Part model, mm, in its own coordinate system. Face numbers are marked on the shaded views. A direction names the side the tool comes from. Give positions to 0.01 mm unless a question says otherwise; leave off trailing zeros. Loops run counter-clockwise (first coordinate to the right, second up) from the corner with the lowest first, then second, coordinate; pieces in that order, holes last. Notation, with made-up numbers: M 89,89.25 L 128,89.25 A29 cw 128,124.25 Z; hole C 29.5,70.25 d9. An arc over 180 degrees is marked long. Put each result on its own line as item: value. Start each with the question number.
Autodesk Inventor part; units mm, degrees
ref_plane "YZ Plane" through (0, 0, 0) normal (1, 0, 0) x (0, 1, 0)
ref_plane "XZ Plane" through (0, 0, 0) normal (0, 1, 0) x (-1, 0, 0)
ref_plane "XY Plane" through (0, 0, 0) normal (0, 0, 1) x (1, 0, 0)
sketch "Sketch1" plane through (0, 0, 0) normal (1, 0, 0) x (0, 1, 0)
  line L0 (16, 0) -> (-16, 0)
  line L1 (16, 0) -> (-16, 0) construction
  line L2 (21.5, 0) -> (16, 0)
  line L3 (21.9436, -96.7485) -> (36.9412, -122.057)
  line L4 (21.5, -4) -> (21.5, -95.1299)
  line L5 (21.5, -95.1299) -> (21.9436, -96.7485)
  line L6 (37.5, -124.0962) -> (37.5, -137.065)
  line L7 (36.9412, -122.057) -> (37.5, -123)
  line L8 (37.5, -123) -> (37.5, -124.0962)
  arc A0 (37.5, -124.0962) -> (36.9412, -122.057) centre (33.5, -124.0962) ccw construction
  line L9 (-16, 0) -> (-20.5, 0)
  line L10 (-20.5, 0) -> (-20.5, -95.1299)
  line L11 (-20.5, -95.1299) -> (-20.5, -4) construction
  line L12 (-20.5, -7.5) -> (-159.2, -7.5)
  line L13 (-159.2, -7.5) -> (-159.2, -52.5)
  line L14 (-159.2, -52.5) -> (-20.5, -52.5)
  line L15 (-73.4, -7.5) -> (-107.4, -7.5) construction
  line L16 (-73.4, -52.5) -> (-107.4, -52.5) construction
  line L17 (-159.2, -35.5) -> (-159.2, -24.5) construction
  line L18 (-35.9412, -122.057) -> (-20.9436, -96.7485)
  line L19 (-20.5, -95.1299) -> (-20.9436, -96.7485)
  line L20 (-36.5, -137.065) -> (-36.5, -124.0962)
  arc A1 (-35.9412, -122.057) -> (-36.5, -124.0962) centre (-32.5, -124.0962) ccw construction
  line L21 (-35.9412, -122.057) -> (-36.5, -123)
  line L22 (-36.5, -123) -> (-36.5, -124.0962)
  line L23 (-36.5, -137.065) -> (-36.5, -141)
  line L24 (-36.5, -141) -> (37.5, -141)
  line L25 (37.5, -141) -> (37.5, -137.065)
  line L26 (-36.5, -139.095) -> (-36.5, -141) construction
  line L27 (37.5, -141) -> (37.5, -139.095) construction
  line L28 (-33.325, -141) -> (34.325, -141) construction
  line L29 (21.5, 0) -> (21.5, -4)
  point P0 (0, 0)
  point P1 (0, 0)
  point P2 (21.5, -10)
  point P3 (16, 0)
  point P4 (-20.5, -52.5)
extrude "Extrusion3" add sketch "Sketch1" along normal mid plane 49
properties part number "BaseBoundingBox"
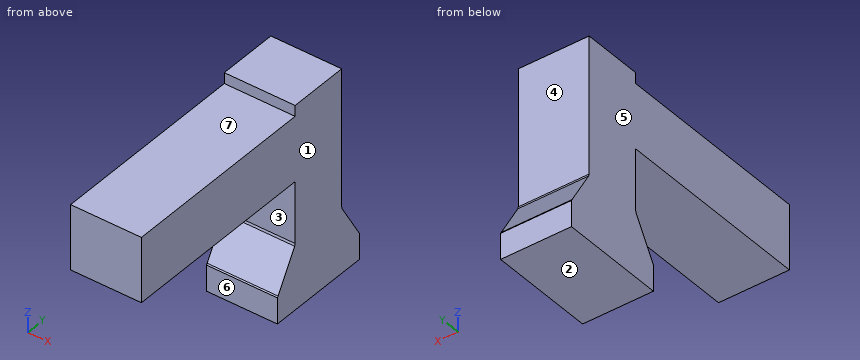
1) Band-saw the part on B-B on x = -1. Give the cut face in (y, z), then the cut area to 3 significant figures.
2) Band-saw the part on A-A on y = -28. Give the cut face in (x, z), then the cut area to 3 significant figures.
3) Band-saw the part on C-C on z = -127. Give the cut face in (x, y), then the cut area to 3 significant figures.
4) Wall check: L1, parallel to Y at x = -17, z = -37.5; L2, parallel to Z at x = 15, y = -122; L3, parallel to Y at x = -21.5, z = -68. Give the ranges that are in metal, low to high.
5) Which spindle directions (+Z, -Z, +X, -X, +Y, -Y) get a long thin tool onto all of the face, cutting with end or side? Do the marked faces 4, 5, 6 and 7. Say none if no direction does.
6) Band-saw the part on D-D on y = -92.5. Give the cut face in (x, z).
7) Mould opens along Z. For the marked faces 1, 2 and 3 say: +Z half, -Z half, draft (parallel to the pull), parting line (faces both ways), or undercut.
8) Pin check, flat tips, straight feed: pin 1 Ø20 at (x, z) = (1.5, -130.5) entering from -Y; pin 2 Ø6 at (x, z) = (-1, -5) entering from -Y; pin 3 Ø14.5 at (x, y) = (11, -117) entering from -Z; pin 4 Ø12 at (x, z) = (-10, -32.5) entering from +Y. Stop position of each tip, or through.
Evaluation:
1. outline: M -159.2,-52.5 L -20.5,-52.5 L -20.5,-95.13 L -20.94,-96.75 L -35.94,-122.06 L -36.5,-123 L -36.5,-141 L 37.5,-141 L 37.5,-123 L 36.94,-122.06 L 21.94,-96.75 L 21.5,-95.13 L 21.5,0 L -20.5,0 L -20.5,-7.5 L -159.2,-7.5 Z
1. area: 13,200 mm2
2. outline: M -24.5,-141 L 24.5,-141 L 24.5,-108.66 L -24.5,-108.66 Z; M -24.5,-52.5 L 24.5,-52.5 L 24.5,-7.5 L -24.5,-7.5 Z
2. area: 3,790 mm2
3. outline: M -24.5,-36.5 L 24.5,-36.5 L 24.5,37.5 L -24.5,37.5 Z
3. area: 3,630 mm2
4. L1: -159.2 to 21.5
4. L2: -52.5 to -7.5
4. L3: -20.5 to 21.5
5. face 4: +Z, +X, -X, +Y
5. face 5: +Z, -Z, -X, +Y, -Y
5. face 6: -Z, +X, -X, -Y
5. face 7: +Z, +X, -X, -Y
6. outline: M -24.5,-52.5 L 24.5,-52.5 L 24.5,-7.5 L -24.5,-7.5 Z
7. face 1: draft
7. face 2: -Z half
7. face 3: undercut
8. pin 1: y = -36.5
8. pin 2: y = -159.2
8. pin 3: z = -52.5
8. pin 4: y = 21.5
